```python
from build123d import *

# Parameters (mm, degrees)
SKETCH2_W = 10
SKETCH2_H = 13.40221624


with BuildPart() as part:
    # Sketch2 → Revolve1 (revolve)
    with BuildSketch(Plane.XY, mode=Mode.PRIVATE) as revolve1_sk:
        Polygon((14, 34.5), (5, 33.40221624), (-5, 33.40221624), (-14, 34.5), (-14, 37.5), (14, 37.5), align=None)
        with Locations((0, 26.70110812)):
            Rectangle(SKETCH2_W, SKETCH2_H)
        Polygon((20, 15), (20, 12), (-20, 12), (-20, 15), (-5, 20), (5, 20), align=None)
    revolve(revolve1_sk.sketch.rotate(Axis((-33.658224077, 0, 0), (1, 0, 0)), 90), axis=Axis((-33.658224077, 0, 0), (1, 0, 0)))


solid = part.part
```
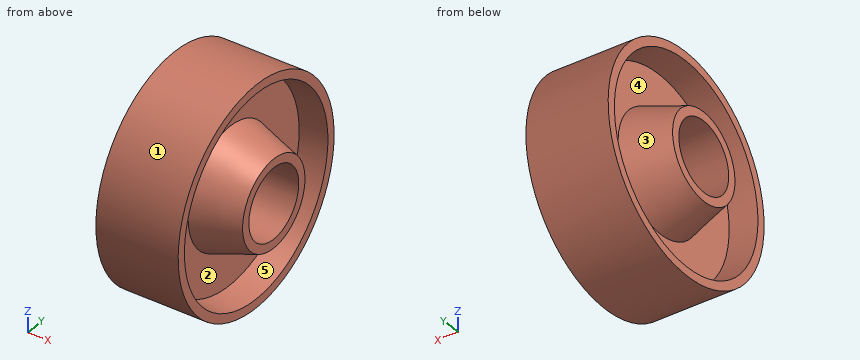
Input: part model. Units: mm. Frame: model coordinates. Face numbers are marked on the shaded views. A direction names the side the tool comes from. Give positions to 0.01 mm unless a question says otherwise; leave off trailing zeros. Write each loop counter-clockwise with the first axis right and the second up, starting at its lowest first coordinate (ties: lowest second). Pieces come first, ordered by that corner, then holes. Notation, with made-up numbers: (87.5, 20.25) - (138.5, 20.25) arc R21 cw to (138.5, 39.25) - close; hole circle Ø1 at (79.25, -32). An arc over 180 degrees is marked (long way). Write item = value, one per line. Start each with the question number.
1) Material intervals for L1, parallel to Y at x = -6, z = -0.5; L2, parallel to Y at x = -13.5, z = 0; L3, parallel to X at y = -17, z = 13.5, sorted ascending. Write a range as [from, to].
2) Pin query (flat end, axial travel): pin 1 (2 mm diameter, centred on x = 8, z = -23.5, fed in from -Y); pin 2 (5 mm diameter, centred on x = -9, z = 20.5, fed in from -Y); pin 3 (5 mm diameter, centred on x = -5, y = -26.5, fed in from +Z). Return the tip coordinate at first contact, or that it passes through.
3) Reachability of the marked faces 4 and 5 from +Z, -Z, +X, -X, +Y, -Y: full face, straight path, thin tool, end or side. Return the list, or none.
4) Cut plane A-A (z = 0). Return loops of the section in (x, y), and give its area (3 significant figures).
5) Draft query along Z for the marked faces 1, 2 and 3. Return one class per face: pulls with the +Z half, pulls with the -Z half, needs draft (parallel to the pull), parting line crosses it, or undercut.
6) Cut plane C-C (x = 3). Return loops of the section in (y, z), and give its area (3 significant figures).
Answers follow:
q1.L1 = [-37.5, -33.52], [-19.66, -11.99], [11.99, 19.66], [33.52, 37.5]
q1.L2 = [-37.5, -34.44], [-17.17, -12], [12, 17.17], [34.44, 37.5]
q1.L3 = [-5, 5]
q2.pin_1 = -30
q2.pin_2 = -32.9
q2.pin_3 = 28.81
q3.face_4 = -X
q3.face_5 = +X
q4.outline = (-20, -15) - (-5, -20) - (-5, -33.4) - (-14, -34.5) - (-14, -37.5) - (14, -37.5) - (14, -34.5) - (5, -33.4) - (5, -20) - (20, -15) - (20, -12) - (-20, -12) - close; (-20, 12) - (20, 12) - (20, 15) - (5, 20) - (5, 33.4) - (14, 34.5) - (14, 37.5) - (-14, 37.5) - (-14, 34.5) - (-5, 33.4) - (-5, 20) - (-20, 15) - close
q4.area = 968 mm^2
q5.face_1 = parting line crosses it
q5.face_2 = undercut
q5.face_3 = undercut
q6.outline = circle Ø75 at (0, 0); hole circle Ø24 at (0, 0)
q6.area = 3,970 mm^2
